Design review of the part built by this model. Coordinates are the model's own, in mm. Give positions to 0.01 mm unless a question says otherwise; leave off trailing zeros. Order: outer loops, then holes, each group sorted by start corner. A loop starts at its lowest first (then second) coordinate and runs counter-clockwise, first axis right, second up.
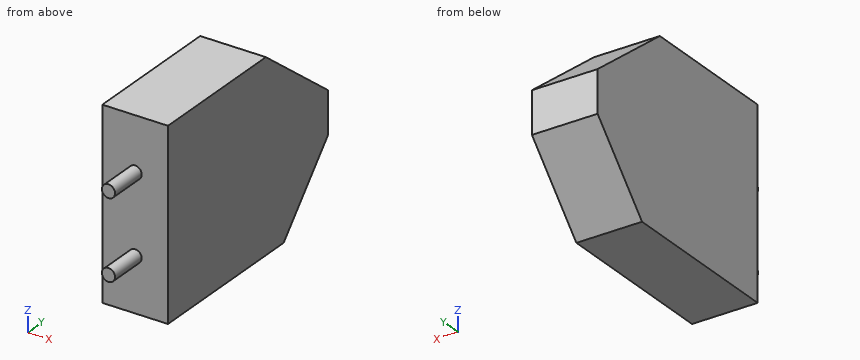
```python
from build123d import *

# Parameters (mm, degrees)
SKETCH_1_W          = 5
SKETCH_1_H          = 14.2
EXTRUDE_1_DEPTH     = 18
SKETCH_2_R          = 0.5
EXTRUDE_2_DEPTH     = 3
CUT_EXTRUDE_1_DEPTH = 5


with BuildPart() as part:
    # 草图1 → 拉伸1 (new body)
    with BuildSketch(Plane(origin=(0, 0, 0), x_dir=(1, 0, 0), z_dir=(0, 1, 0))):
        Rectangle(SKETCH_1_W, SKETCH_1_H)
    extrude(amount=EXTRUDE_1_DEPTH)

    # 草图2 → 拉伸2 (add)
    with BuildSketch(Plane.XZ):
        with Locations(Location((0, 3, 0), (0, 0, 90))):
            Circle(SKETCH_2_R)
        with Locations(Location((0, -3, 0), (0, 0, 90))):
            Circle(SKETCH_2_R)
    extrude(amount=EXTRUDE_2_DEPTH)

    # 草图3 → 切除-拉伸1 (cut)
    with BuildSketch(Plane(origin=(2.5, 0, 0), x_dir=(0, 0, -1), z_dir=(1, 0, 0))):
        Polygon((-1.6, 18), (-7.1, 11), (-7.1, 18), align=None)
        Polygon((1.6, 18), (7.1, 13), (7.1, 18), align=None)
    extrude(amount=-CUT_EXTRUDE_1_DEPTH, mode=Mode.SUBTRACT)


solid = part.part
```
1. Take a section at B-B (z = -1). State the section outline as (x, y) points.
Recorded:
outline: (-2.5, 0) - (2.5, 0) - (2.5, 18) - (-2.5, 18) - close
2. Take a section at C-C (x = 0). State the section outline as (y, z) points, then the cut area to 3 significant figures.
Recorded:
outline: (-3, -3.5) - (0, -3.5) - (0, -7.1) - (13, -7.1) - (18, -1.6) - (18, 1.6) - (11, 7.1) - (0, 7.1) - (0, 3.5) - (-3, 3.5) - (-3, 2.5) - (0, 2.5) - (0, -2.5) - (-3, -2.5) - close
area: 229 mm2
3. Take a section at D-D (y = 16). State the section outline as (x, z) points, then the cut area to 3 significant figures.
Recorded:
outline: (-2.5, -3.8) - (2.5, -3.8) - (2.5, 3.17) - (-2.5, 3.17) - close
area: 34.9 mm2
4. For pin 1 (1 mm diameter, centred on x = 1, z = -2, fed in from -Y), flat-tipped, find the tip position at first contact; note if it passes through.
Recorded:
pin 1: stops at y = 0
5. For line 1 along Y through (x, z) = (2.1, -1.5); line 2 along Y through (x, z) = (1.95, -6); line 3 along Z through (x, y) = (1.4, 14), list the stretches that pass through material, from the lowest coordinate up.
Recorded:
line 1: y = 0 to 18
line 2: y = 0 to 14
line 3: z = -6 to 4.74
6. Take a section at A-A (x = -1.15). State the section outline as (y, z) points, then the cut area to 3 significant figures.
Recorded:
outline: (0, -7.1) - (13, -7.1) - (18, -1.6) - (18, 1.6) - (11, 7.1) - (0, 7.1) - close
area: 223 mm2
